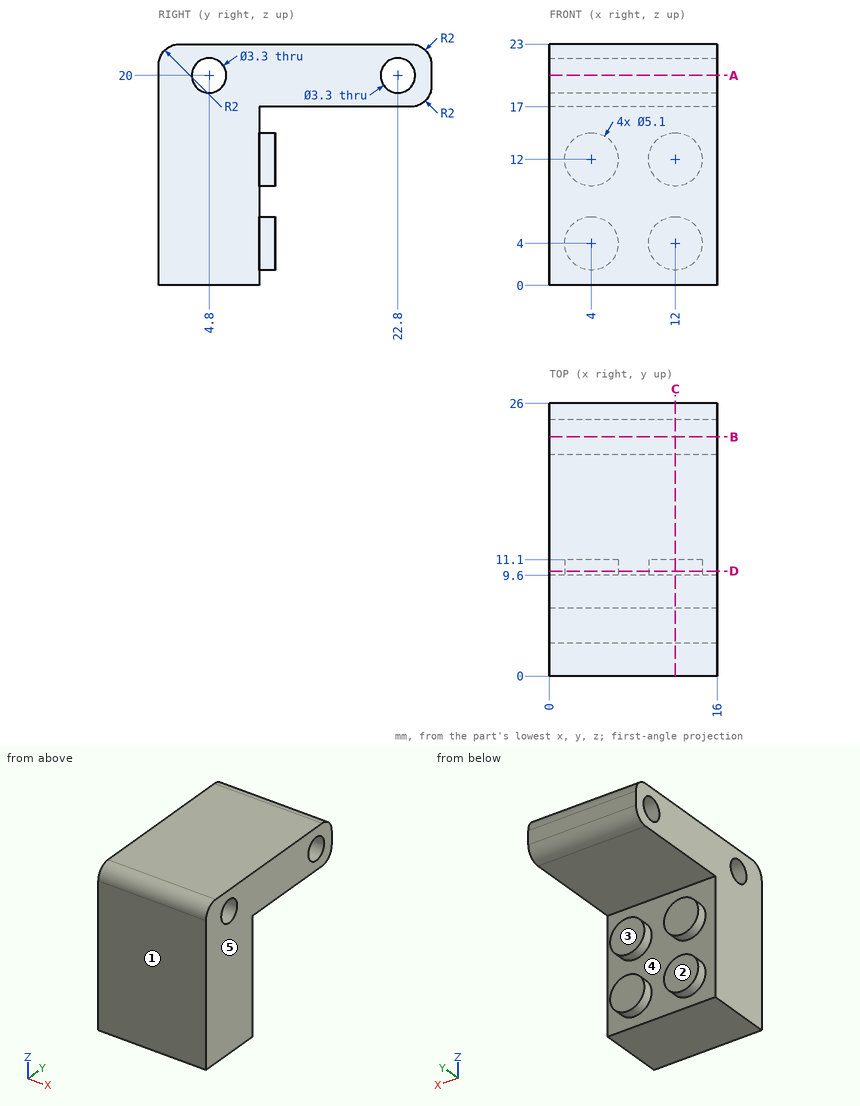
Study the drawing (mm; zero at the part's minimum x, y, z) and answer. A direction names the side the tool comes from. Give positions to 0.01 mm unless a question says otherwise; leave off trailing zeros. Order: outer loops, then holes, each group sorted by start corner. A loop starts at its lowest first (then second) coordinate and runs counter-clockwise, first axis right, second up. Notation, with made-up numbers: (0.5, 24.25) - (40.5, 24.25) arc R22 cw to (40.5, 45.25) - close; hole circle Ø6 at (-3, 6). An arc over 180 degrees is marked (long way). Use one line per item in the form item = value. Start each with the question number.
(1) A cutting plane is placed at D-D, the plane y = 10. Write down the section's boundary in (x, z).
(2) Consider line 1 (Z direction, x = 8, y = 22.8); line 2 (Z direction, x = 8.75, y = 4.8); line 3 (Z direction, x = 12.75, y = 14.5). Determine where each line is inside the solid, lowest interval first. Write a range as from..to.
(3) A cutting plane is placed at C-C, the plane x = 12. Write down the section's boundary in (y, z), then the cut area to 3 significant figures.
(4) A cutting plane is placed at A-A, the plane z = 20. Write down the section's boundary in (x, y), then the cut area to 3 significant figures.
(5) Flat-ended cylindrical pins translate along their axes: pin 1 Ø2 at (y, z) = (22.8, 20) entering from -X; pin 2 Ø1.5 at (x, z) = (4.5, 11) entering from +Y; pin 3 Ø5 at (x, y) = (1.5, 14) entering from -Z. Find the tip coordinate at first contact, or state that the pin passes through.
(6) The mould has two halves that part along X. Classify the marked faces 3, 4 and 5: released by +X, released by -X, zero draft, split by the parting line, or undercut.
(7) A cutting plane is placed at B-B, the plane y = 22.8. Write down the section's boundary in (x, z).
(8) For the marked faces 1 and 2, determine the directions among +Z, -Z, +X, -X, +Y, -Y from which every point of the face is accessible in a straight line to the end or side of a thin tool.
Ans:
q1.outline = (0, 17) - (16, 17) - (16, 23) - (0, 23) - close; circle Ø5.1 at (4, 4); circle Ø5.1 at (4, 12); circle Ø5.1 at (12, 4); circle Ø5.1 at (12, 12)
q2.line_1 = 17..18.35, 21.65..23
q2.line_2 = 0..18.35, 21.65..23
q2.line_3 = 17..23
q3.outline = (0, 0) - (9.6, 0) - (9.6, 1.45) - (11.1, 1.45) - (11.1, 6.55) - (9.6, 6.55) - (9.6, 9.45) - (11.1, 9.45) - (11.1, 14.55) - (9.6, 14.55) - (9.6, 17) - (24, 17) arc R2 ccw to (26, 19) - (26, 21) arc R2 ccw to (24, 23) - (2, 23) arc R2 ccw to (0, 21) - close; hole circle Ø3.3 at (4.8, 20); hole circle Ø3.3 at (22.8, 20)
q3.area = 315 mm^2
q4.outline = (0, 0) - (16, 0) - (16, 3.15) - (0, 3.15) - close; (0, 6.45) - (16, 6.45) - (16, 21.15) - (0, 21.15) - close; (0, 24.45) - (16, 24.45) - (16, 26) - (0, 26) - close
q4.area = 310 mm^2
q5.pin_1 = through
q5.pin_2 = 11.1
q5.pin_3 = 17
q6.face_3 = zero draft
q6.face_4 = undercut
q6.face_5 = released by +X
q7.outline = (0, 17) - (16, 17) - (16, 18.35) - (0, 18.35) - close; (0, 21.65) - (16, 21.65) - (16, 23) - (0, 23) - close
q8.face_1 = +Z, -Z, +X, -X, -Y
q8.face_2 = -Z, +X, -X, +Y
